Here's the drawing with two shaded views (mm, measured from the low corner). I have some questions. A direction names the side the tool comes from. Give positions to 0.01 mm unless a question says otherwise; leave off trailing zeros. Order: outer loops, then holes, each group sorted by start corner. A loop starts at its lowest first (then second) coordinate and runs counter-clockwise, first axis right, second up. Notation, with made-up numbers: M -31,68 L 22,68 A34 ccw 22,104 Z; hole C 43,58 d8. An arc over 180 degrees is marked long. Use a Markdown table: item, result. Add a question column.
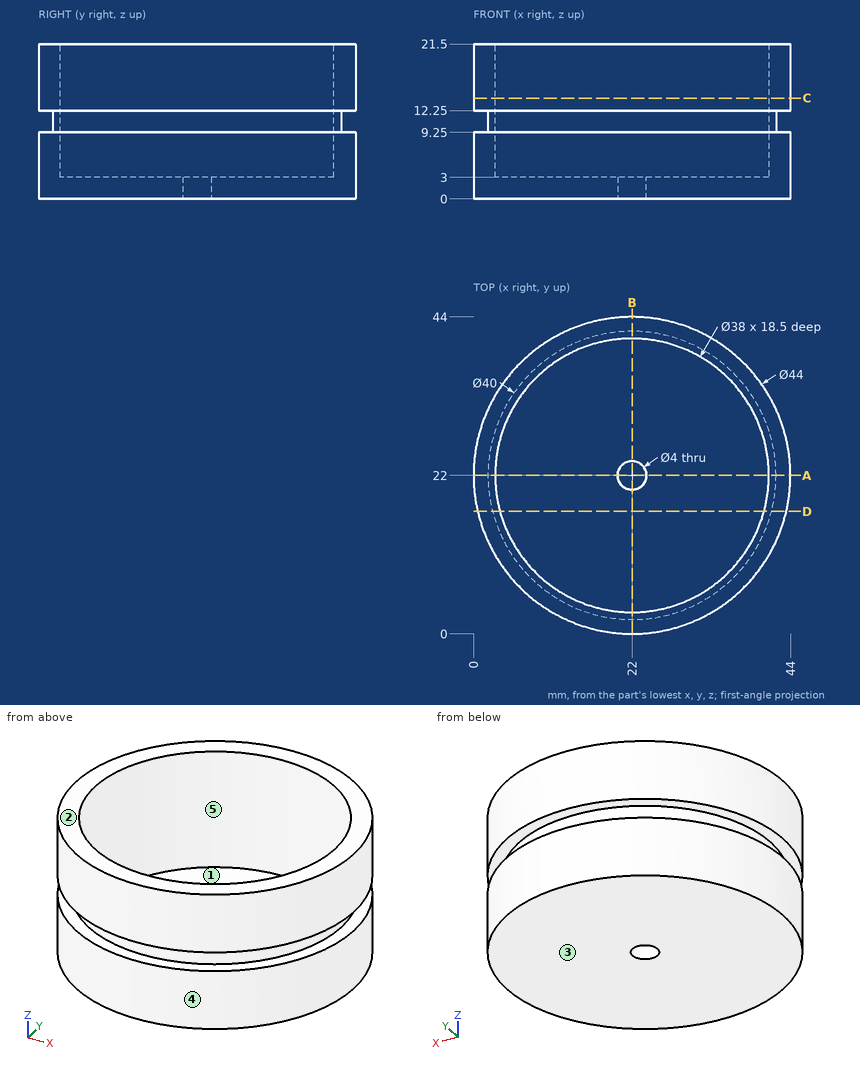
1. If we section it at A-A, the plane y = 22: List the corners of the cut face in (x, z) for me.
2. Will these pins go through, and if not, where does the flat tip stop? pin 1 (3 mm diameter, centred on x = 28, z = 17, fed in from +Y); pin 2 (6 mm diameter, centred on y = 4.5, z = 4, fed in from +X); pin 3 (8 mm diameter, centred on y = 15, z = 15.5, fed in from -X).
3. If we section it at D-D, the plane y = 17: List the corners of the cut face in (x, z) for me, then the cut area to 3 significant figures.
4. I need wall thicknesses on L1, parallel to Y at x = 22, z = 14.75; L2, parallel to Y at x = 22, z = 1.6; L3, parallel to Z at x = 39, y = 8.5. Which ranges of each line are inside material? Lowest first, please. Write a range as [from, to].
5. We'd pull the mould along X, two halves only. Please class the marked faces 3, 4 and 5: +X half, -X half, draft (parallel to the pull), parting line (faces both ways), or undercut.
6. If we section it at C-C, the plane z = 14: List the corners of the cut face in (x, y) for me, then the cut area to 3 significant figures.
7. On a 3-axis mill with a long thin cutter (end or side, diameter ignored), from which of +Z, -Z, +X, -X, +Y, -Y can I reach the whole of each face in a straight line? I mean the marked faces 1 and 2. Say none if no direction works.
Geometry results:
| question | item | result |
|---|---|---|
| 1 | outline | M 0,0 L 20,0 L 20,3 L 3,3 L 3,21.5 L 0,21.5 L 0,12.25 L 2,12.25 L 2,9.25 L 0,9.25 Z; M 24,0 L 44,0 L 44,9.25 L 42,9.25 L 42,12.25 L 44,12.25 L 44,21.5 L 41,21.5 L 41,3 L 24,3 Z |
| 2 | pin 1 | stops at y = 43.53 |
| 2 | pin 2 | stops at x = 38.55 |
| 2 | pin 3 | stops at x = 0.21 |
| 3 | outline | M 0.58,0 L 43.42,0 L 43.42,9.25 L 41.36,9.25 L 41.36,12.25 L 43.42,12.25 L 43.42,21.5 L 40.33,21.5 L 40.33,3 L 3.67,3 L 3.67,21.5 L 0.58,21.5 L 0.58,12.25 L 2.64,12.25 L 2.64,9.25 L 0.58,9.25 Z |
| 3 | area | 231 mm^2 |
| 4 | L1 | y = [0, 3], [41, 44] |
| 4 | L2 | y = [0, 20], [24, 44] |
| 4 | L3 | z = [0, 9.25], [12.25, 21.5] |
| 5 | face 3 | draft |
| 5 | face 4 | parting line |
| 5 | face 5 | undercut |
| 6 | outline | C 22,22 d44; hole C 22,22 d38 |
| 6 | area | 386 mm^2 |
| 7 | face 1 | +Z |
| 7 | face 2 | +Z, +X, -X, +Y, -Y |
